Design review of the part built by this model. Coordinates are the model's own, in mm. A direction names the side the tool comes from. Coordinates: 2 decimals unless noted, no trailing zeros. Loops run counter-clockwise (first coordinate to the right, second up) from the corner with the lowest first, then second, coordinate; pieces in that order, holes last. Notation, with made-up numbers: (8, -31.5) -> (14, -31.5) arc R21 ccw to (14, -21.5) -> close; hole circle Ø2 at (36, 68.25). An arc over 180 degrees is marked (long way). Answer in a Markdown table with one row per item.
```python
from build123d import *

# Parameters (mm, degrees)
F0_W     = 600
F0_H     = 600
F1_DEPTH = 380
F2_SIZE2 = 202.0725942164
F2_SIZE  = 350
F3_W     = 195.8548115673
F3_H     = 195.8548115673
F4_DEPTH = 440


with BuildPart() as f1:
    # F0 (on Top) → F1 (new body)
    with BuildSketch(Plane.XY):
        with Locations((-300, 300)):
            Rectangle(F0_W, F0_H)
    extrude(amount=F1_DEPTH)

    # F2
    f2_edges = [f1.edges().sort_by_distance(p)[0] for p in [
        (-300, 0, 380),
        (0, 300, 380),
        (-300, 600, 380),
        (-600, 300, 380),
    ]]
    chamfer(f2_edges, length=F2_SIZE, length2=F2_SIZE2)

    # F3 (on face) → F4 (join)
    with BuildSketch(Plane.XY.offset(380)):
        with Locations((-300, 300)):
            Rectangle(F3_W, F3_H)
    extrude(amount=F4_DEPTH)


solid = f1.part
```
(1) To check wall thickness, follow probe 1 along Y at (x, z) = (-248, 408); probe 2 along Z at (x, y) = (-561, 290); probe 3 along Z at (x, y) = (-310, 470.5). State the ranges of each line that lie inside material, in increasing order.
Evaluation:
| item | result |
|---|---|
| probe 1 | y = 202.07 to 397.93 |
| probe 2 | z = 0 to 97.55 |
| probe 3 | z = 0 to 254.3 |
(2) For pin 1 (4 mm diameter, centred on y = 239, z = 614.5, fed in from +X); pin 2 (2 mm diameter, centred on x = -381.5, z = 556, fed in from -Y); pin 3 (6 mm diameter, centred on x = -218, z = 201.5, fed in from +Y), all flat-tipped, find the tip position at first contact; note any pin that passes through.
Evaluation:
| item | result |
|---|---|
| pin 1 | stops at x = -202.07 |
| pin 2 | stops at y = 202.07 |
| pin 3 | stops at y = 502.72 |
(3) Tool access review of faces 1 (the flat face through (-202.073, 299, 597)), 2 (the flat face through (-397.927, 299, 597)), 3 (the flat face through (-301, 202.073, 597)), 4 (the flat face through (-301, 397.927, 597)): name each direction out of +Z, -Z, +X, -X, +Y, -Y from which nothing blocks a thin tool from reaching the whole face with its end or side.
Evaluation:
| item | result |
|---|---|
| face 1 | +Z, +X, +Y, -Y |
| face 2 | +Z, -X, +Y, -Y |
| face 3 | +Z, +X, -X, -Y |
| face 4 | +Z, +X, -X, +Y |
(4) Take a section at A-A on x = -242.5. Give the boundary of the cut face in (y, z).
Evaluation:
| item | result |
|---|---|
| outline | (0, 0) -> (600, 0) -> (600, 30) -> (397.93, 380) -> (397.93, 820) -> (202.07, 820) -> (202.07, 380) -> (0, 30) -> close |
(5) Take a section at B-B on y = 377. Give the boundary of the cut face in (x, z), and give its area (3 significant figures).
Evaluation:
| item | result |
|---|---|
| outline | (-600, 0) -> (0, 0) -> (0, 30) -> (-202.07, 380) -> (-202.07, 820) -> (-397.93, 820) -> (-397.93, 380) -> (-600, 30) -> close |
| area | 243,000 mm² |
(6) Take a section at D-D on y = 495. Give the boundary of the cut face in (x, z), and give its area (3 significant figures).
Evaluation:
| item | result |
|---|---|
| outline | (-600, 0) -> (0, 0) -> (0, 30) -> (-105, 211.87) -> (-495, 211.87) -> (-600, 30) -> close |
| area | 108,000 mm² |
(7) Take a section at C-C on z = 329.5. Give the boundary of the cut face in (x, y), and give its area (3 significant figures).
Evaluation:
| item | result |
|---|---|
| outline | (-427.08, 172.92) -> (-172.92, 172.92) -> (-172.92, 427.08) -> (-427.08, 427.08) -> close |
| area | 64,600 mm² |
